Read the model definition and answer for the solid it produces. Units are mm, in the model's axes. A direction names the side the tool comes from. Coordinates: 2 decimals unless noted, no trailing zeros. Loops run counter-clockwise (first coordinate to the right, second up) from the corner with the lowest first, then second, coordinate; pieces in that order, holes last. Notation, with made-up numbers: (70, 27) -> (114, 27) arc R15 cw to (114, 42) -> close; hole circle Ø10 at (88.5, 51). An arc over 180 degrees is marked (long way). Answer in a Markdown table with one row per item.
```python
from build123d import *

# Parameters (mm, degrees)
F0_W     = 20
F0_H     = 35
F0_H_2   = 40
F1_DEPTH = 20


with BuildPart() as f1:
    # F0 (on Front) → F1 (new body)
    with BuildSketch(Plane.XZ):
        Polygon((89.008551, 73.575356), (-70.991449, 73.575356), (-70.991449, 33.575356), (-70.991449, -1.424644), (-70.991449, -36.424644), (-70.991449, -76.424644), (89.008551, -76.424644), align=None)
        with Locations((-80.991449, 16.075356)):
            Rectangle(F0_W, F0_H)
        with Locations((-80.991449, -56.424644)):
            Rectangle(F0_W, F0_H_2)
    extrude(amount=F1_DEPTH)


solid = f1.part
```
1. A tool of negligible diameter and unlimited length cuts with its end or side. For faces 5 (the flat face through (-70.991, -10, 54)), 6 (the flat face through (-90.991, -10, 16)), 7 (the flat face through (-81, -10, -1.425)), from which of +Z, -Z, +X, -X, +Y, -Y can it reach the whole face along a straight path? Write none if from no direction.
A:
| item | result |
|---|---|
| face 5 | +Z, -X, +Y, -Y |
| face 6 | +Z, -Z, -X, +Y, -Y |
| face 7 | -X, +Y, -Y |
2. A cutting plane is placed at B-B on z = -14. Give the vertices of the cut face in (x, y).
A:
| item | result |
|---|---|
| outline | (-70.99, -20) -> (89.01, -20) -> (89.01, 0) -> (-70.99, 0) -> close |
3. The mould has two halves that part along Z. Classify faces 1 (the flat face through (-2, -20, 0)), 2 (the flat face through (-2, -10, -76.425)), 3 (the flat face through (-81, -10, -36.425)), 4 (the flat face through (10, -10, 73.575)): pulls with the +Z half, pulls with the -Z half, needs draft (parallel to the pull), parting line crosses it, or undercut.
A:
| item | result |
|---|---|
| face 1 | needs draft |
| face 2 | pulls with the -Z half |
| face 3 | undercut |
| face 4 | pulls with the +Z half |
4. Given pin 1 Ø5 at (x, z) = (7.5, -49.5) entering from +Y; pin 2 Ø10 at (y, z) = (-10, 55.5) entering from -X; pin 3 Ø6 at (x, y) = (-83.5, -14.5) entering from +Z, each flat-ended and moving along its own axis, determine where each tip first touches the part or whether it passes through.
A:
| item | result |
|---|---|
| pin 1 | stops at y = 0 |
| pin 2 | stops at x = -70.99 |
| pin 3 | stops at z = 33.58 |
5. A cutting plane is placed at A-A on y = -2.25. Give the vertices of the cut face in (x, z).
A:
| item | result |
|---|---|
| outline | (-90.99, -76.42) -> (89.01, -76.42) -> (89.01, 73.58) -> (-70.99, 73.58) -> (-70.99, 33.58) -> (-90.99, 33.58) -> (-90.99, -1.42) -> (-70.99, -1.42) -> (-70.99, -36.42) -> (-90.99, -36.42) -> close |
6. Find the intervals of material crossed by probe 1 along X at (y, z) = (-5.75, -2), in increasing order.
A:
| item | result |
|---|---|
| probe 1 | x = -70.99 to 89.01 |
